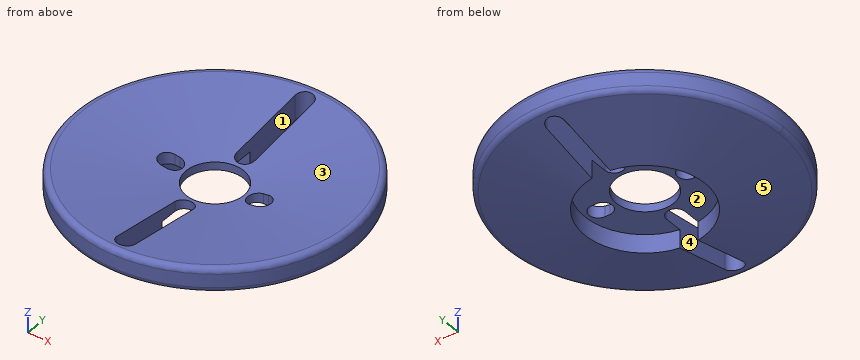
from build123d import *

# Parameters (mm, degrees)
SKETCH1_R           = 26.5
SKETCH1_R_2         = 5.5
BOSS_EXTRUDE1_DEPTH = 1.5
HOLES_DEPTH         = 38.7458607
FILLET2_R           = 1
HOLES_PTR_COUNT     = 2


with BuildPart() as part:
    # Sketch1 → Boss-Extrude1 (new body)
    with BuildSketch(Plane.XY):
        Circle(SKETCH1_R)
        Circle(SKETCH1_R_2, mode=Mode.SUBTRACT)
    extrude(amount=BOSS_EXTRUDE1_DEPTH)

    # Sketch8 → Revolve2 (revolve)
    with BuildSketch(Plane(origin=(0, 0, 0), x_dir=(1, 0, 0), z_dir=(0, 1, 0))):
        Polygon((-11.5, 0), (-11.5, 3.5), (-26.5, 0), align=None)
        Polygon((5.5, -1.5), (26.5, -1.5), (26.5, -4.5), align=None)
    revolve(axis=Axis((0, 0, 0), (0, 0, 1)))

    # Sketch7 → holes (cut, symmetric)
    with BuildSketch(Plane.XY):
        with BuildLine():
            Line((1.75, -8), (1.75, -23))
            ThreePointArc((1.75, -23), (0, -24.75), (-1.75, -23))
            Line((-1.75, -23), (-1.75, -8))
            ThreePointArc((-1.75, -8), (0, -6.25), (1.75, -8))
        make_face()
        with BuildLine():
            Line((8, 1.75), (9, 1.75))
            ThreePointArc((9, 1.75), (10.75, 0), (9, -1.75))
            Line((9, -1.75), (8, -1.75))
            ThreePointArc((8, -1.75), (6.25, 0), (8, 1.75))
        make_face()
    holes = extrude(amount=HOLES_DEPTH, both=True, mode=Mode.SUBTRACT)

    # Fillet2
    fillet2_edges = [part.edges().sort_by_distance(p)[0] for p in [
        (0, 26.5, 0),
        (-26.5, 0, 4.5),
    ]]
    fillet(fillet2_edges, radius=FILLET2_R)

    # holes-ptr: holes ×2 about axis
    holes_ptr_axis = Axis((0, 0, 0), (0, 0, 1))
    for i in range(1, HOLES_PTR_COUNT):
        add(holes.rotate(holes_ptr_axis, i * 360 / HOLES_PTR_COUNT), mode=Mode.SUBTRACT)


solid = part.part
Model file for the job. Use its own axes, mm. Face numbers are marked on the shaded views. A direction names the side the tool comes from. Give positions to 0.01 mm unless a question says otherwise; leave off trailing zeros. Use one line per item in the form item = value.
(1) 3-axis set-ups, long thin cutter, end or side, ignore diameter. For the marked faces 1, 2 and 3: which of +Z, -Z, +X, -X, +Y, -Y reach the whole face in a straight line?
Determined:
face_1 = +Z, -Z
face_2 = -Z
face_3 = +Z
(2) Drill centre lines: L1, parallel to Y at x = 0, z = 1.1; L2, parallel to Y at x = 0, z = 0.4; L3, parallel to X at y = 12, z = 1. Where is each one in solid material? Low to high.
Determined:
L1 = -26.5 to -24.75, -6.25 to -5.5, 5.5 to 6.25, 24.75 to 26.5
L2 = -26.42 to -24.75, -6.25 to -5.5, 5.5 to 6.25, 24.75 to 26.42
L3 = -23.63 to -1.75, 1.75 to 23.63
(3) Pull direction Y, two halves, no side cores. Call the marked faces 4 and 5: pulls with the +Y half, pulls with the -Y half, needs draft (parallel to the pull), parting line crosses it, or undercut.
Determined:
face_4 = undercut
face_5 = parting line crosses it
(4) Drop flat-ended pins along their axis: P1, Ø0.8, axis at x = -8.5, z = 1, coming from the -Y side; P2, Ø4, axis at y = -13.5, z = -1.5, coming from the +X side; P3, Ø1.5, axis at x = 14.5, z = 2.5, coming from the -Y side. Give the stop position or say it passes through.
Determined:
P1 = -25.23
P2 = 23.17
P3 = -22.65
